Design review of the part built by this model. Coordinates are the model's own, in mm. A direction names the side the tool comes from. Give positions to 0.01 mm unless a question says otherwise; leave off trailing zeros. Write each loop counter-clockwise with the first axis right and the second up, starting at its lowest first coordinate (ties: lowest second). Pieces come first, ordered by that corner, then holes.
```python
from build123d import *

# Parameters (mm, degrees)
F0_R     = 2
F1_DEPTH = 6
F2_R     = 4.4
F3_DEPTH = 4
F4_R     = 3.5
F4_R_2   = 2.75
F5_DEPTH = 7
F6_W     = 13
F6_H     = 6
F7_DEPTH = 23
F9_DEPTH = 10


with BuildPart() as f1:
    # F0 (on Front) → F1 (new body)
    with BuildSketch(Plane.XZ):
        with BuildLine():
            Line((0, 3), (32.554146, 0))
            Line((32.554146, 0), (61.188469, 0))
            Line((61.188469, 0), (63.609742, 0))
            ThreePointArc((63.609742, 0), (65.29669, 4.018384), (68.75, 1.359841))
            ThreePointArc((68.75, 1.359841), (68.658544, 0.65653), (68.390258, 0))
            Line((68.390258, 0), (70.811531, 0))
            Line((70.811531, 0), (113, 0))
            Line((113, 0), (115.5, 0))
            ThreePointArc((115.5, 0), (119, 3.5), (122.5, 0))
            Line((122.5, 0), (125, 0))
            Line((125, 0), (125, 1.644468))
            ThreePointArc((125, 1.644468), (124.341818, 4.124108), (122.540554, 5.950927))
            Line((122.540554, 5.950927), (117.372112, 9))
            Line((117.372112, 9), (0, 9))
            Line((0, 9), (0, 3))
        make_face()
        with Locations((46, 4.333029)):
            Circle(F0_R, mode=Mode.SUBTRACT)
        with Locations((89, 4.333029)):
            Circle(F0_R, mode=Mode.SUBTRACT)
        with BuildLine():
            Line((63.609742, 0), (61.188469, 0))
            ThreePointArc((61.188469, 0), (66, -3.640159), (70.811531, 0))
            Line((70.811531, 0), (68.390258, 0))
            ThreePointArc((68.390258, 0), (66, -1.390159), (63.609742, 0))
        make_face()
        with BuildLine():
            ThreePointArc((0, 9), (-3, 6), (0, 3))
            Line((0, 3), (0, 9))
        make_face()
        with BuildLine():
            Line((115.5, 0), (113, 0))
            ThreePointArc((113, 0), (119, -6), (125, 0))
            Line((125, 0), (122.5, 0))
            ThreePointArc((122.5, 0), (119, -3.5), (115.5, 0))
        make_face()
    extrude(amount=F1_DEPTH)

    # F2 (on face) → F3 (cut)
    with BuildSketch(Plane(origin=(0, 0, 0), x_dir=(-1, 0, 0), z_dir=(0, 1, 0))):
        with Locations((-119, 0)):
            Circle(F2_R)
    extrude(amount=-F3_DEPTH, mode=Mode.SUBTRACT)

    # F4 (on face) → F5 (join)
    with BuildSketch(Plane(origin=(0, 0, 0), x_dir=(-1, 0, 0), z_dir=(0, 1, 0))):
        with Locations((-66, 1.359841)):
            Circle(F4_R)
        with Locations((-66, 1.359841)):
            Circle(F4_R_2, mode=Mode.SUBTRACT)
    extrude(amount=-F5_DEPTH)

    # F6 (on face) → F7 (join)
    with BuildSketch(Plane.XZ.offset(6)):
        with BuildLine():
            Line((0, 3), (0, 9))
            ThreePointArc((0, 9), (-3, 6), (0, 3))
        make_face()
        with Locations((6.5, 6)):
            Rectangle(F6_W, F6_H)
        with BuildLine():
            ThreePointArc((13, 3), (16, 6), (13, 9))
            Line((13, 9), (13, 3))
        make_face()
    extrude(amount=F7_DEPTH)

    # F8 (on face) → F9 (join)
    with BuildSketch(Plane.XZ.offset(29)):
        with BuildLine():
            Line((13, 7.7), (-0.358373, 7.661797))
            ThreePointArc((-0.358373, 7.661797), (-1.7, 6), (-0.358373, 4.338203))
            Line((-0.358373, 4.338203), (13, 4.3))
            ThreePointArc((13, 4.3), (14.7, 6), (13, 7.7))
        make_face()
    extrude(amount=F9_DEPTH)


solid = f1.part
```
(1) Clearance check with flat-ended pins moving along their axes: P1, Ø7.5, axis at x = 39.5, z = -0.5, coming from the -Y side; P2, Ø6.5, axis at x = 81.5, y = -3.5, coming from the -Z side; P3, Ø6.5, axis at x = 3.5, y = -12.5, coming from the -Z side. State where each tip first meets the part, or that it passes through.
Resolved:
P1: stops at y = -6
P2: stops at z = 0
P3: stops at z = 3
(2) To check wall thickness, follow L1, parallel to X at y = -2, z = 4.5; L2, parallel to Z at x = 66, y = -4.4; L3, parallel to Z at x = 35.5, y = -3. State the ranges of each line that lie inside material, in increasing order.
Resolved:
L1: x = -2.6 to 44.01, 47.99 to 87.01, 90.99 to 124.1
L2: z = -3.64 to -1.39, 4.11 to 9
L3: z = 0 to 9
(3) Consider section C-C, the plane x = 46. Give the boundary of the cut face in (y, z).
Resolved:
outline: (-6, 0) - (0, 0) - (0, 2.33) - (-6, 2.33) - close; (-6, 6.33) - (0, 6.33) - (0, 9) - (-6, 9) - close
(4) Consider section B-B, the plane y = -2.5. Give the boundary of the cut face in (x, z).
Resolved:
outline: (0, 3) - (32.55, 0) - (61.19, 0) arc R5 ccw to (70.81, 0) - (113, 0) arc R6 ccw to (125, 0) - (125, 1.64) arc R5 ccw to (122.54, 5.95) - (117.37, 9) - (0, 9) arc R3 ccw to start; hole circle Ø4 at (46, 4.33); hole circle Ø5.5 at (66, 1.36); hole circle Ø4 at (89, 4.33); hole circle Ø8.8 at (119, 0)
(5) Tool access review of faces 5 (the face through (6, -39, 6)), 6 (the face through (92, -3, 0)), 7 (the face through (47, -3, 0)), 8 (the face through (14.7, -33.9, 6)), 9 (the face through (68.6, -6.5, 3.7)): name each direction out of +Z, -Z, +X, -X, +Y, -Y from which nothing blocks a thin tool from reaching the whole face with its end or side.
Resolved:
face 5: +Z, -Z, +X, -X, -Y
face 6: -Z, +Y, -Y
face 7: -Z, -X, +Y, -Y
face 8: +X, -Y
face 9: -Y
(6) Mouldability with a two-part tool opening along Z and no side actions: class faces 1 (the face through (114.936, -1.972, -1.685)), 2 (the face through (-1.7, -33.9, 6)), 3 (the face through (119.993, -2.958, 7.454)), 4 (the face through (119, -4, -4)) as pulls with the +Z half, pulls with the -Z half, needs draft (parallel to the pull), parting line crosses it, or undercut.
Resolved:
face 1: undercut
face 2: parting line crosses it
face 3: pulls with the +Z half
face 4: undercut
(7) Consider section A-A, the plane x = 66. Give the boundary of the cut face in (y, z), then the cut area to 3 significant figures.
Resolved:
outline: (-7, -2.14) - (-6, -2.14) - (-6, -3.64) - (0, -3.64) - (0, -1.39) - (-7, -1.39) - close; (-7, 4.11) - (0, 4.11) - (0, 9) - (-6, 9) - (-6, 4.86) - (-7, 4.86) - close
area: 44.3 mm2
(8) Consider section D-D, the plane y = -31.5. Give the boundary of the cut face in (x, z).
Resolved:
outline: (-0.36, 4.34) - (13, 4.3) arc R1.7 ccw to (13, 7.7) - (-0.36, 7.66) arc R1.7 ccw to start
